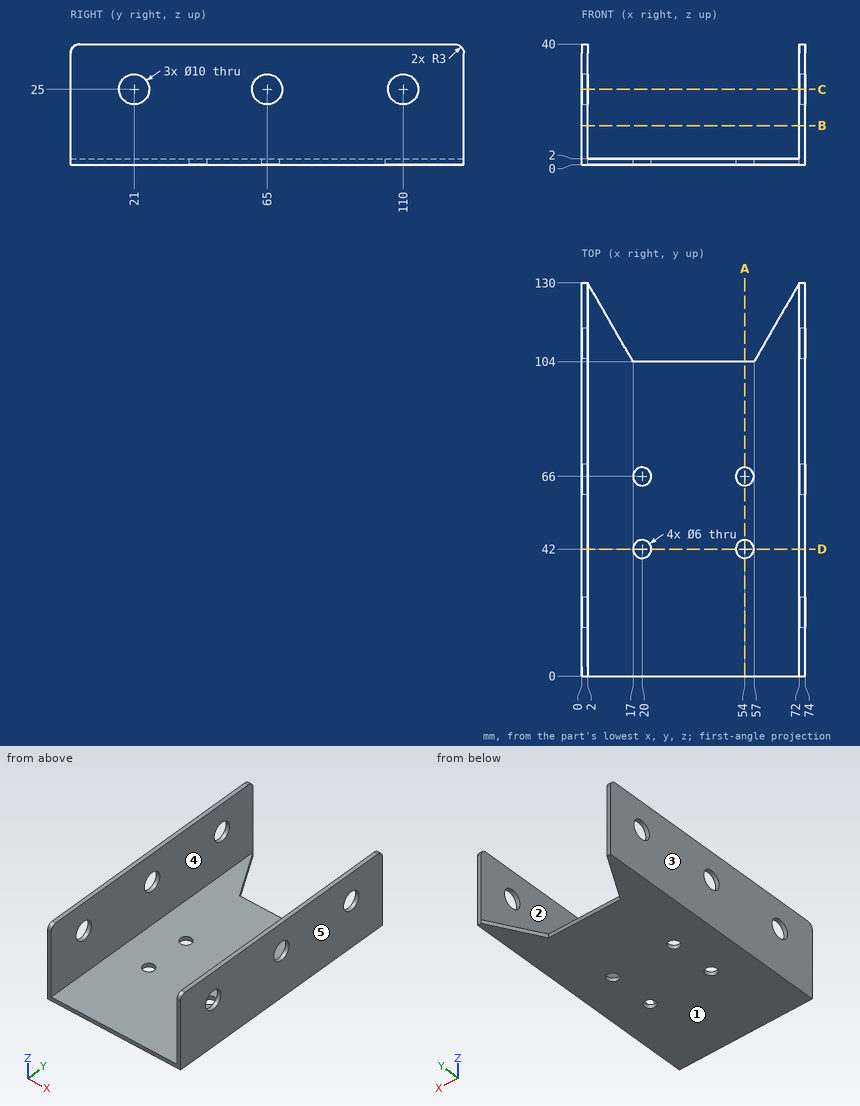
Verification items for this drawing (mm, ordinates from the low corner). A direction names the side the tool comes from. Give positions to 0.01 mm unless a question says otherwise; leave off trailing zeros. Loops run counter-clockwise (first coordinate to the right, second up) from the corner with the lowest first, then second, coordinate; pieces in that order, holes last. Notation, with made-up numbers: M 54.25,-24 L 111.25,-24 A22 cw 111.25,10 Z; hole C 60,-1.75 d10. An arc over 180 degrees is marked long. Write item = value, one per line.
(1) Sectioned sample at A-A, the plane x = 54. Record the cut outline in (y, z), plus the area to 3 significant figures.
Answer below:
outline = M 0,0 L 39,0 L 39,2 L 0,2 Z; M 45,0 L 63,0 L 63,2 L 45,2 Z; M 69,0 L 104,0 L 104,2 L 69,2 Z
area = 184 mm2
(2) Gauge pin test, flat ends, axial feed: pin 1 Ø21 at (x, y) = (21, 35.5) entering from +Z; pin 2 Ø2 at (x, z) = (34, 0.5) entering from +Y. Record the tip position at first contact, or that the pin passes through.
Answer below:
pin_1 = 2
pin_2 = 104
(3) Tool access check on the marked faces 4 and 5. Record the directions out of +Z, -Z, +X, -X, +Y, -Y that give a thin tool (end or side, any length) a straight path to the whole face; none if there is none.
Answer below:
face_4 = +Z, +Y, -Y
face_5 = +Z, -Z, +X, +Y, -Y
(4) Sectioned sample at D-D, the plane y = 42. Record the cut outline in (x, z).
Answer below:
outline = M 0,0 L 17,0 L 17,2 L 2,2 L 2,40 L 0,40 Z; M 23,0 L 51,0 L 51,2 L 23,2 Z; M 57,0 L 74,0 L 74,40 L 72,40 L 72,2 L 57,2 Z
(5) Release check for a two-part mould opening along X. For the marked faces 1, 2 and 3 record: released by +X, released by -X, zero draft, split by the parting line, or undercut.
Answer below:
face_1 = zero draft
face_2 = undercut
face_3 = released by -X
(6) Sectioned sample at C-C, the plane z = 25. State how many separate pieces and enclosed holes the cut face has, plus the area to 3 significant figures.
Answer below:
separate_pieces = 8
enclosed_holes = 0
area = 400 mm2
(7) Material ranges on line 1 (Y direction, x = 73.3, z = 25); line 2 (X direction, y = 84, z = 14.5); line 3 (Z direction, x = 51, y = 84.5), recorded low to high. Write a range as [from, to].
Answer below:
line_1 = [0, 16], [26, 60], [70, 105], [115, 130]
line_2 = [0, 2], [72, 74]
line_3 = [0, 2]
(8) Sectioned sample at B-B, the plane z = 13. Record the cut outline in (x, y), plus the area to 3 significant figures.
Answer below:
outline = M 0,0 L 2,0 L 2,130 L 0,130 Z; M 72,0 L 74,0 L 74,130 L 72,130 Z
area = 520 mm2
